Print and shaded views of the part. All mm, measured from the part's lowest x, y and z. A direction names the side the tool comes from. Coordinates: 2 decimals unless noted, no trailing zeros. Loops run counter-clockwise (first coordinate to the right, second up) from the corner with the lowest first, then second, coordinate; pieces in that order, holes last. Notation, with made-up numbers: (81, 71.25) -> (89, 71.25) arc R22 ccw to (89, 91.25) -> close; hole circle Ø9 at (59.5, 6.25). An arc over 180 degrees is marked (long way). One line per item, written item: value. Start each with the question number.
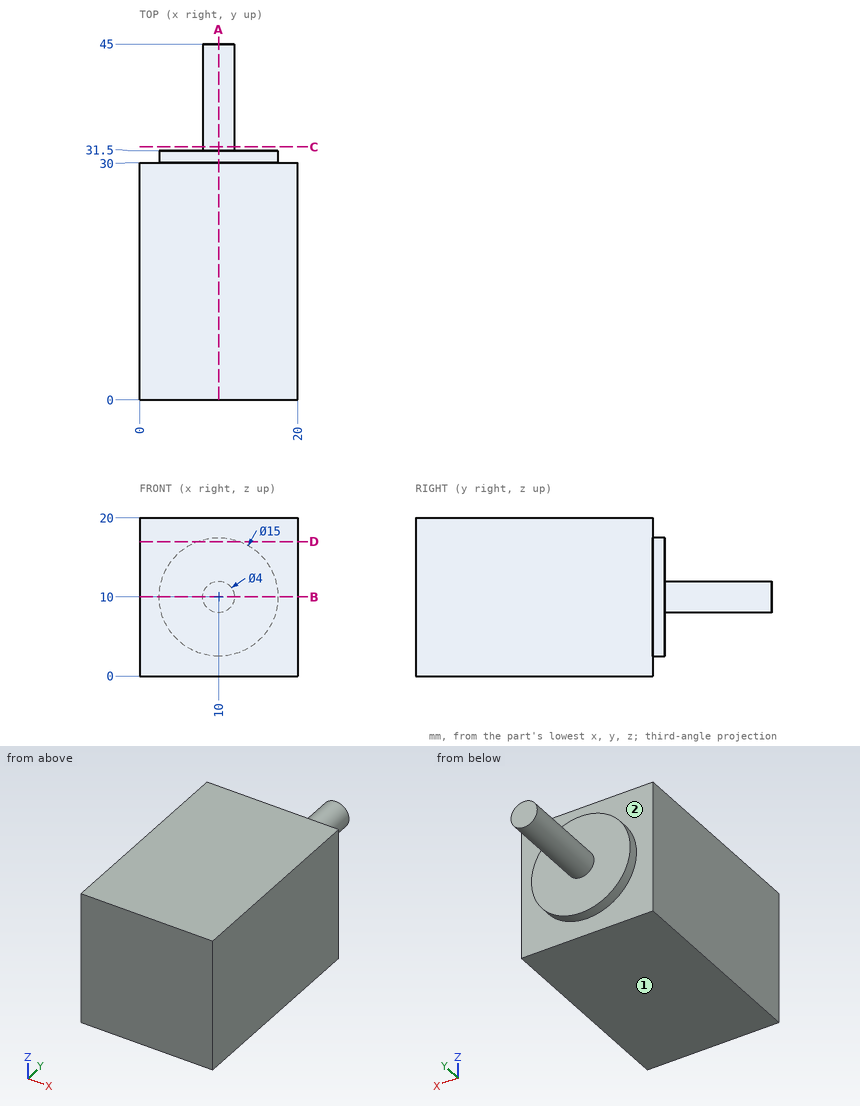
1) Slice it at D-D (z = 17). Give the cut face in (x, y), then the cut area to 3 significant figures.
2) Tool access for the marked faces 1 and 2: list every direction of +Z, -Z, +X, -X, +Y, -Y with a clear straight run to the whole face (end or side of a thin tool).
3) Slice it at A-A (x = 10). Give the cut face in (y, z).
4) Slice it at B-B (z = 10). Give the cut face in (x, y), then the cut area to 4 significant figures.
5) Slice it at C-C (y = 32). Give the cut face in (x, z).
6) Pin check, flat tip, straight feed: pin 1 Ø1.5 at (y, z) = (39.5, 12) entering from +X. Stop position of the tip, or through.
7) Probe line 1 (Y direction, x = 10.5, z = 7.75); line 2 (Y direction, x = 3.5, z = 6); line 3 (X direction, y = 30.5, z = 15.75). List the from-to ranges inside material, lowest first. Write a range as from..to.
Check sheet entries:
1. outline: (0, 0) -> (20, 0) -> (20, 30) -> (12.69, 30) -> (12.69, 31.5) -> (7.31, 31.5) -> (7.31, 30) -> (0, 30) -> close
1. area: 608 mm^2
2. face 1: -Z, +X, -X, +Y, -Y
2. face 2: +Y
3. outline: (0, 0) -> (30, 0) -> (30, 2.5) -> (31.5, 2.5) -> (31.5, 8) -> (45, 8) -> (45, 12) -> (31.5, 12) -> (31.5, 17.5) -> (30, 17.5) -> (30, 20) -> (0, 20) -> close
4. outline: (0, 0) -> (20, 0) -> (20, 30) -> (17.5, 30) -> (17.5, 31.5) -> (12, 31.5) -> (12, 45) -> (8, 45) -> (8, 31.5) -> (2.5, 31.5) -> (2.5, 30) -> (0, 30) -> close
4. area: 676.5 mm^2
5. outline: circle Ø4 at (10, 10)
6. pin 1: stops at x = 11.56
7. line 1: y = 0..31.5
7. line 2: y = 0..30
7. line 3: x = 5.18..14.82
